```python
from build123d import *

# Parameters (mm, degrees)
F0_W     = 200
F0_H     = 100
F1_DEPTH = 100
F2_R     = 36.887858
F3_DEPTH = 50


with BuildPart() as f1:
    # F0 (on Front) → F1 (new body)
    with BuildSketch(Plane.XZ):
        Rectangle(F0_W, F0_H)
    extrude(amount=-F1_DEPTH)

    # F2 (on face) → F3 (join)
    with BuildSketch(Plane.XY.offset(50)):
        with Locations((0, 47.454495)):
            Circle(F2_R)
    extrude(amount=F3_DEPTH)


solid = f1.part
```
Work out the finished part from the listing and answer in its coordinate system (mm). A direction names the side the tool comes from. Give positions to 0.01 mm unless a question says otherwise; leave off trailing zeros. Loops run counter-clockwise (first coordinate to the right, second up) from the corner with the lowest first, then second, coordinate; pieces in that order, holes last. Notation, with made-up numbers: M 16.5,-33 L 58.5,-33 A27 cw 58.5,-3 Z; hole C 61,12.5 d7. An arc over 180 degrees is marked long. One line per item, written item: value. Start each with the question number.
1. Find the intervals of material crossed by probe 1 along Z at (x, y) = (67.5, 20); probe 2 along X at (y, z) = (49, 70); probe 3 along X at (y, z) = (68.5, 55), in increasing order.
2. Find section C-C (x = -50.5). Give the vertices of the cut face in (y, z).
3. Find section A-A (x = 0). Give the vertices of the cut face in (y, z), and give its area (3 significant figures).
4. Each of these flat-tipped pins is pushed along its axis until it touches: P1, Ø8, axis at y = 14.5, z = 55, coming from the -X side (3 decimals); P2, Ø5, axis at y = 38, z = 72, coming from the -X side. Where does it stop, or does it pass through?
5. Which of the six approach directions +Z, -Z, +X, -X, +Y, -Y give full straight-line access (tool end or side, diameter ignored) to faces 1 (the face through (-1, 49, -50)), 2 (the face through (19.83, 78.56, 74.65))?
6. Find section B-B (y = 30). Give the vertices of the cut face in (x, z), and give its area (3 significant figures).
Reported:
1. probe 1: z = -50 to 50
1. probe 2: x = -36.86 to 36.86
1. probe 3: x = -30.3 to 30.3
2. outline: M 0,-50 L 100,-50 L 100,50 L 0,50 Z
3. outline: M 0,-50 L 100,-50 L 100,50 L 84.34,50 L 84.34,100 L 10.57,100 L 10.57,50 L 0,50 Z
3. area: 13,700 mm²
4. P1: stops at x = -22.855
4. P2: stops at x = -36.23
5. face 1: -Z, +X, -X, +Y, -Y
5. face 2: +Z
6. outline: M -100,-50 L 100,-50 L 100,50 L 32.5,50 L 32.5,100 L -32.5,100 L -32.5,50 L -100,50 Z
6. area: 23,200 mm²
